Geometry: see drawing. Coordinates: mm, zero at the bounding-box minimum. Round coordinates to 2 decimals unless told otherwise and drop trailing zeros. Write each loop counter-clockwise with the first axis right and the second up, starting at its lowest first coordinate (ties: lowest second). Pieces come first, ordered by that corner, then holes. Notation, with made-up numbers: M 42.25,64 L 82.25,64 A21 cw 82.25,82 Z; hole C 64.25,29.25 d10. An arc over 180 degrees is marked long. Use a Markdown table: item, result.
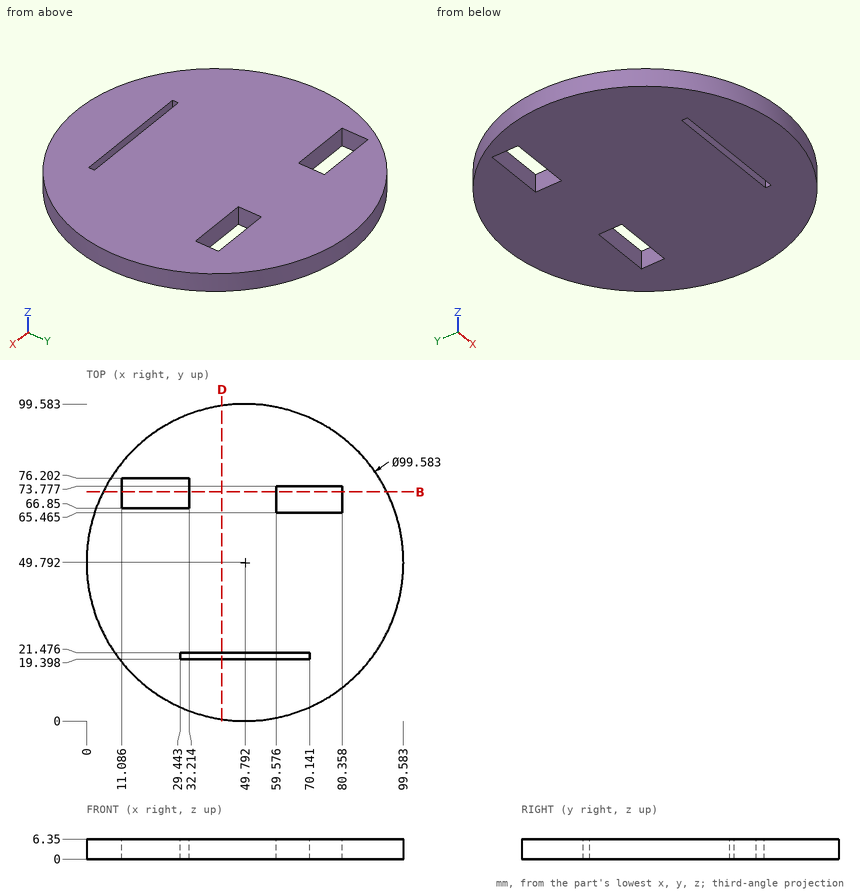
Q1. Section B-B on y = 72. Give the number of separate pieces and of enclosed holes in the cut face, plus the area to 3 significant figures.
Results are:
| item | result |
|---|---|
| separate pieces | 3 |
| enclosed holes | 0 |
| area | 300 mm^2 |
Q2. Section D-D on x = 42.5. Return loops of the section in (y, z).
Results are:
| item | result |
|---|---|
| outline | M 0.54,0 L 19.4,0 L 19.4,6.35 L 0.54,6.35 Z; M 21.48,0 L 99.05,0 L 99.05,6.35 L 21.48,6.35 Z |
Q3. Line query: L1, parallel to X at y = 72, z = 5.5 (1 decimal); L2, parallel to Y at x = 57.5, z = 2.75; L3, parallel to X at y = 74, z = 3 (1 decimal). Output: solid intervals per line, ascending.
Results are:
| item | result |
|---|---|
| L1 | 5.2 to 11.1, 32.2 to 59.6, 80.4 to 94.4 |
| L2 | 0.6 to 19.4, 21.48 to 98.98 |
| L3 | 6.3 to 11.1, 32.2 to 93.3 |
Q4. First-contact query: pin 1 Ø3 at (y, z) = (69.5, 4.5) entering from -X; pin 2 Ø1 at (y, z) = (20.5, 2.5) entering from +X (1 decimal); pin 3 Ø1 at (y, z) = (11, 1) entering from -X (1 decimal). Flat tips, straight axial feed; report the tip coordinate or a pass-through.
Results are:
| item | result |
|---|---|
| pin 1 | x = 3.45 |
| pin 2 | x = 90.4 |
| pin 3 | x = 18 |
